Autodesk Inventor part; units mm, degrees
ref_plane "YZ Plane" through (0, 0, 0) normal (1, 0, 0) x (0, 1, 0)
ref_plane "XZ Plane" through (0, 0, 0) normal (0, 1, 0) x (-1, 0, 0)
ref_plane "XY Plane" through (0, 0, 0) normal (0, 0, 1) x (1, 0, 0)
sketch "Sketch1" plane through (0, 0, 0) normal (0, 1, 0) x (-1, 0, 0)
  circle A0 centre (0, 0) radius 17.5
  dimension "d0" = 35
extrude "Extrusion1" add sketch "Sketch1" along normal blind 8
fillet "Fillet1" radius 2 1 edges at (17.5, 8, 0)
sketch "Sketch2" plane through (0, 8, 0) normal (0, 1, 0) x (1, 0, 0)
  point P0 (0, 0)
  point P1 (0, 0)
hole "Hole1" at (0, 8, 0) direction (0, -1, 0) diameter 14.5 end through all countersink diameter 25 countersink angle 90
sketch "Sketch3" plane through (0, 8, 0) normal (0, 1, 0) x (1, 0, 0)
  point P0 (0, 0)
properties part number "washer.special" material "Steel, High Strength, Low Alloy"
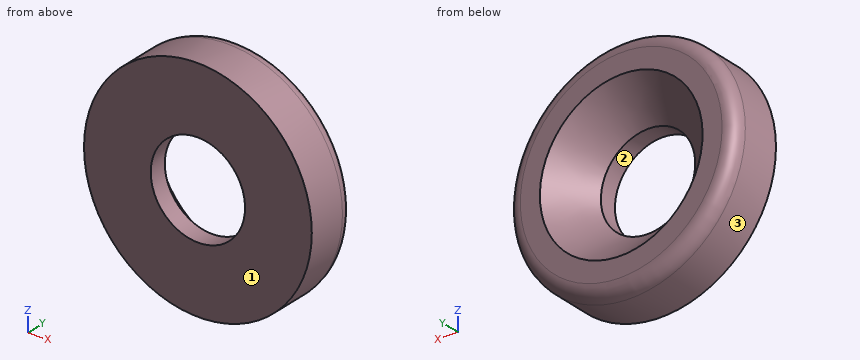
Geometry check sheet. Reference: the model listing, model coordinates, mm. Face numbers are marked on the shaded views. Round coordinates to 2 decimals unless told otherwise and drop trailing zeros. Loops run counter-clockwise (first coordinate to the right, second up) from the corner with the lowest first, then second, coordinate; pieces in that order, holes last. Notation, with made-up numbers: (47.5, 7.25) - (98.5, 7.25) arc R30 cw to (98.5, 46.25) - close; hole circle Ø11 at (71, 80). An arc over 180 degrees is marked (long way). Answer as CSV lines item,"result".
(1) Material ranges on line 1 along Z through (x, y) = (0, 1.15); line 2 along X through (y, z) = (2.5, 3); line 3 along Z through (x, y) = (7, 6), recorded low to high.
Output values:
line 1,"z = -17.5 to -7.25, 7.25 to 17.5"
line 2,"x = -17.24 to -6.6, 6.6 to 17.24"
line 3,"z = -16.04 to -7.83, 7.83 to 16.04"
(2) Depth check by flat-ended pin: pin 1 Ø4 at (y, z) = (5, -7) entering from +X; pin 2 Ø3 at (x, y) = (-9.5, 2.5) entering from -Z; pin 3 Ø4 at (x, y) = (6.5, 1) entering from +Z. Enter the tip coordinate at first touch or a pass-through.
Output values:
pin 1,"stops at x = 16.77"
pin 2,"stops at z = -15.56"
pin 3,"stops at z = 16.91"
(3) Cross-section at C-C, the plane y = 2. Enter the section's corners in (x, z).
Output values:
outline,"circle Ø35 at (0, 0); hole circle Ø14.5 at (0, 0)"
(4) Cross-section at D-D, the plane y = 5.25. Enter the section's corners in (x, z), and give its area (3 significant figures).
Output values:
outline,"circle Ø35 at (0, 0); hole circle Ø19.5 at (0, 0)"
area,"663 mm²"
(5) Cross-section at B-B, the plane x = 0. Enter the section's corners in (y, z), and give its area (3 significant figures).
Output values:
outline,"(0, -17.5) - (6, -17.5) arc R2 ccw to (8, -15.5) - (8, -12.5) - (2.75, -7.25) - (0, -7.25) - close; (0, 7.25) - (2.75, 7.25) - (8, 12.5) - (8, 15.5) arc R2 ccw to (6, 17.5) - (0, 17.5) - close"
area,"135 mm²"
(6) Release check for a two-part mould opening along Z. For the marked faces 1, 2 and 3 record: released by +Z, released by -Z, zero draft, split by the parting line, or undercut.
Output values:
face 1,"zero draft"
face 2,"undercut"
face 3,"split by the parting line"
(7) Cross-section at A-A, the plane z = 0. Enter the section's corners in (x, y), and give its area (3 significant figures).
Output values:
outline,"(-17.5, 0) - (-7.25, 0) - (-7.25, 2.75) - (-12.5, 8) - (-15.5, 8) arc R2 ccw to (-17.5, 6) - close; (7.25, 0) - (17.5, 0) - (17.5, 6) arc R2 ccw to (15.5, 8) - (12.5, 8) - (7.25, 2.75) - close"
area,"135 mm²"
